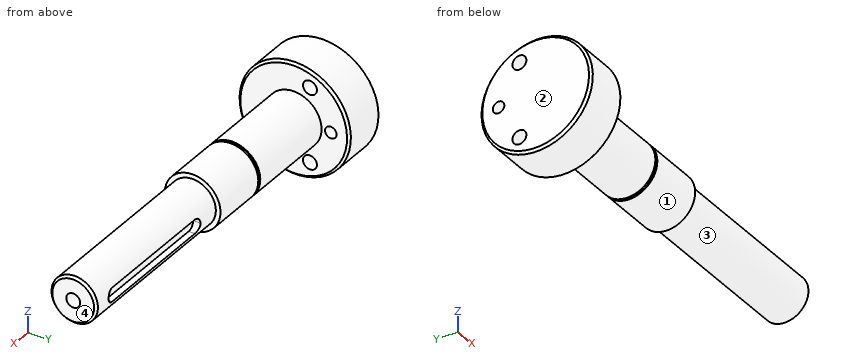
from build123d import *

# Parameters (mm, degrees)
PER_AGE1_D              = 5
PER_AGE1_DEPTH          = 17
PER_AGE1_CBORE_D        = 6
PER_AGE1_CBORE_DEPTH    = 12
PER_AGE1_TIP            = 1.502151548
ESQUISSE6_W             = 1.3
ESQUISSE6_H             = 0.5
ESQUISSE5_W             = 60
ESQUISSE5_H             = 3.145636389
ENL_V_MAT_EXTRU_1_DEPTH = 3
CONG_1_R                = 3
CHANFREIN1_SIZE         = 1
ESQUISSE7_R             = 3
ESQUISSE7_R_2           = 2.5
ENL_V_MAT_EXTRU_2_DEPTH = 168.475371324


with BuildPart() as part:
    # Esquisse1 → Base-Révolution (revolve)
    with BuildSketch(Plane.XY, mode=Mode.PRIVATE) as base_r_volution_sk:
        Polygon((0, 0), (0, 24), (20, 24), (20, 12), (86, 12), (86, 10), (164, 10), (164, 0), align=None)
    revolve(base_r_volution_sk.sketch.rotate(Axis((0, 0, 0), (1, 0, 0)), 90), axis=Axis((0, 0, 0), (1, 0, 0)))

    # Perçage1
    with Locations(Plane(origin=(164, 0, 0), x_dir=(0, 0, -1), z_dir=(1, 0, 0))):
        with Locations((0, 0)):
            CounterBoreHole(PER_AGE1_D / 2, PER_AGE1_CBORE_D / 2, PER_AGE1_CBORE_DEPTH, depth=PER_AGE1_DEPTH)
            with Locations((0, 0, -(PER_AGE1_DEPTH + PER_AGE1_TIP / 2))):  # 118° drill point
                Cone(0, PER_AGE1_D / 2, PER_AGE1_TIP, mode=Mode.SUBTRACT)

    # Esquisse6 → Enlèvement de matière-Révolution1 (revolve, cut)
    with BuildSketch(Plane.XY, mode=Mode.PRIVATE) as enl_vement_de_mati_re_r_volution1_sk:
        with Locations((60.65, 11.75)):
            Rectangle(ESQUISSE6_W, ESQUISSE6_H)
    revolve(enl_vement_de_mati_re_r_volution1_sk.sketch.rotate(Axis((0, 0, 0), (1, 0, 0)), 90), axis=Axis((0, 0, 0), (1, 0, 0)), mode=Mode.SUBTRACT)

    # Esquisse5 → Enlèv. mat.-Extru.1 (cut, symmetric)
    with BuildSketch(Plane.XY):
        with Locations((126, 8.427181806)):
            Rectangle(ESQUISSE5_W, ESQUISSE5_H)
    extrude(amount=ENL_V_MAT_EXTRU_1_DEPTH, both=True, mode=Mode.SUBTRACT)

    # Congé1
    cong_1_edges = [part.edges().sort_by_distance(p)[0] for p in [
        (96, 8.196877813, 3),
        (156, 8.196877813, 3),
        (156, 8.196877813, -3),
        (96, 8.196877813, -3),
    ]]
    fillet(cong_1_edges, radius=CONG_1_R - 0.0001)  # a hair under: the kernel refuses the full size

    # Chanfrein1
    chanfrein1_edges = [part.edges().sort_by_distance(p)[0] for p in [
        (164, 0, -10),
        (20, 0, -24),
        (0, 0, -24),
    ]]
    chamfer(chanfrein1_edges, length=CHANFREIN1_SIZE)

    # Esquisse7 → Enlèv. mat.-Extru.2 (cut, through all)
    with BuildSketch(Plane.ZY):
        with Locations((-16, 7)):
            Circle(ESQUISSE7_R)
        with Locations((16, 7)):
            Circle(ESQUISSE7_R)
        with Locations((0, 16)):
            Circle(ESQUISSE7_R_2)
    extrude(amount=-ENL_V_MAT_EXTRU_2_DEPTH, mode=Mode.SUBTRACT)


solid = part.part
Source: CAD feature listing. Evaluate the final solid. Frame: model axes, mm. Face numbers are marked on the shaded views. A direction names the side the tool comes from. Give positions to 0.01 mm unless a question says otherwise; leave off trailing zeros. Write item = value, one per line.
Item 1: Ray query, probe 1 along Y at (x, z) = (6.5, 0); probe 2 along Y at (x, z) = (149, 0); probe 3 along X at (y, z) = (-14, 2). Return the intervals inside material, ascending.
Check result:
probe_1 = -24 to 13.5, 18.5 to 24
probe_2 = -10 to -2.5, 2.5 to 6.85
probe_3 = 0 to 20
Item 2: Set-up query: the marked faces 3 and 4. Return all of +Z, -Z, +X, -X, +Y, -Y with unobstructed straight access to the full face (end or side cutting, diameter ignored); none if empty.
Check result:
face_3 = +X
face_4 = +Z, -Z, +X, +Y, -Y
Item 3: Contact query for flat-ended pins moving along their axis: pin 1 (3 mm diameter, centred on x = 129, y = 8.5, fed in from +Z); pin 2 (5 mm diameter, centred on x = 80.5, y = -8.5, fed in from -Z); pin 3 (0.8 mm diameter, centred on x = 119, y = 8.5, fed in from -Z). Output: stop coordinate, or through.
Check result:
pin_1 = 7.14
pin_2 = -10.39
pin_3 = -5.86
Item 4: Mould query, pull axis Z, two halves, no side actions, for the marked faces 1 and 2. Classes: +Z half, -Z half, draft (parallel to the pull), parting line (faces both ways), or undercut.
Check result:
face_1 = parting line
face_2 = draft
